Geometry: see drawing. Coordinates: mm, zero at the bounding-box minimum. Coordinates: 2 decimals unless noted, no trailing zeros. Write each loop counter-clockwise with the first axis right and the second up, starting at its lowest first coordinate (ties: lowest second). Pieces come first, ordered by that corner, then holes.
1) Pin query (flat end, axial travel): pin 1 Ø4 at (x, z) = (116.5, 250) entering from -Y. Return the tip coordinate at first contact, or that it passes through.
2) Section query C-C (y = 3.25). Output: boundary loops of the cut face in (x, z), then the cut area to 3 significant figures.
3) Line query: L1, parallel to Z at x = 225, y = 10.5; L2, parallel to X at y = 7.75, z = 250; L3, parallel to X at y = 6, z = 93.5. Output: solid intervals per line, ascending.
4) Section query A-A (x = 75). Output: boundary loops of the cut face in (y, z).
5) Section query B-B (z = 50). Output: boundary loops of the cut face in (x, y).
6) Section query D-D (x = 143). Output: boundary loops of the cut face in (y, z).
7) Draft query along X for the marked faces 1 and 2. Return one class per face: pulls with the +X half, pulls with the -X half, needs draft (parallel to the pull), parting line crosses it, or undercut.
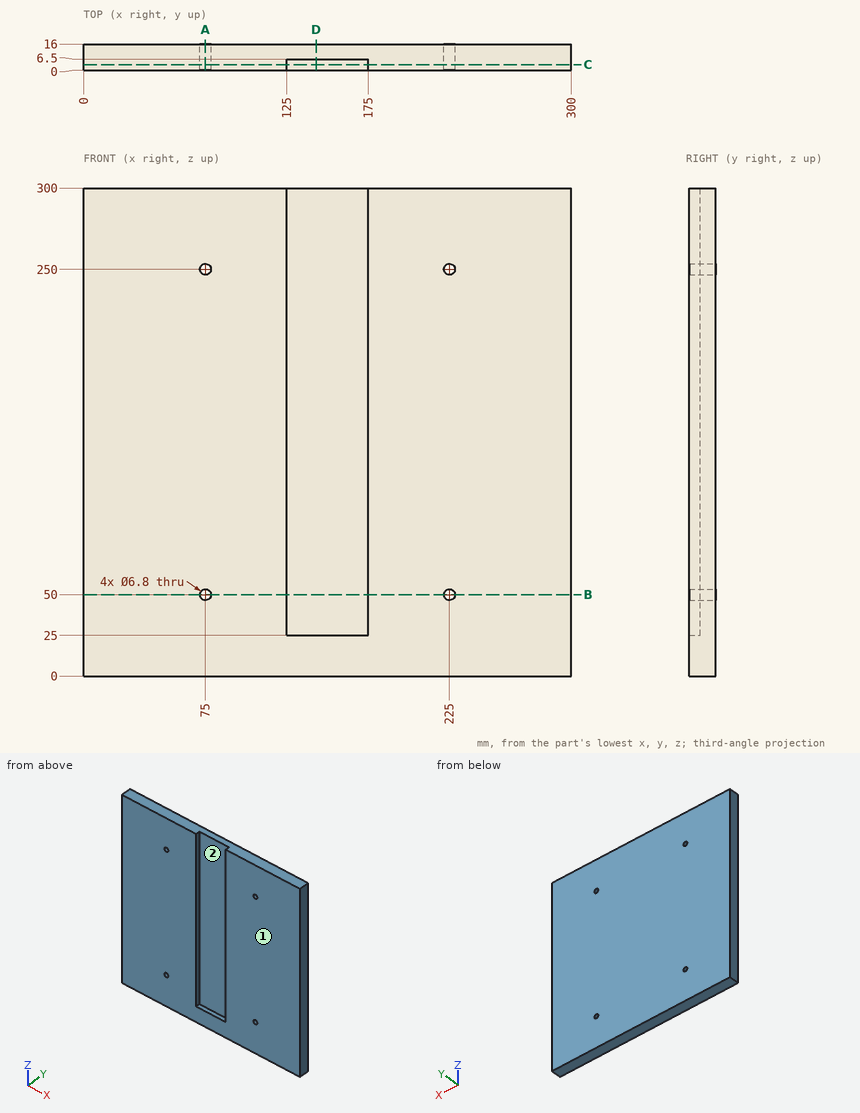
Answer:
1. pin 1: stops at y = 0
2. outline: (0, 0) - (300, 0) - (300, 300) - (175, 300) - (175, 25) - (125, 25) - (125, 300) - (0, 300) - close; hole circle Ø6.8 at (75, 50); hole circle Ø6.8 at (75, 250); hole circle Ø6.8 at (225, 50); hole circle Ø6.8 at (225, 250)
2. area: 76,100 mm2
3. L1: z = 0 to 46.6, 53.4 to 246.6, 253.4 to 300
3. L2: x = 0 to 71.6, 78.4 to 221.6, 228.4 to 300
3. L3: x = 0 to 125, 175 to 300
4. outline: (0, 0) - (16, 0) - (16, 46.6) - (0, 46.6) - close; (0, 53.4) - (16, 53.4) - (16, 246.6) - (0, 246.6) - close; (0, 253.4) - (16, 253.4) - (16, 300) - (0, 300) - close
5. outline: (0, 0) - (71.6, 0) - (71.6, 16) - (0, 16) - close; (78.4, 0) - (125, 0) - (125, 6.5) - (175, 6.5) - (175, 0) - (221.6, 0) - (221.6, 16) - (78.4, 16) - close; (228.4, 0) - (300, 0) - (300, 16) - (228.4, 16) - close
6. outline: (0, 0) - (16, 0) - (16, 300) - (6.5, 300) - (6.5, 25) - (0, 25) - close
7. face 1: needs draft
7. face 2: undercut
